For this review, use the dimensioned drawing (mm, ordinates from the lowest corner) and the shaded views. A direction names the side the tool comes from. Coordinates: 2 decimals unless noted, no trailing zeros. Loops run counter-clockwise (first coordinate to the right, second up) from the corner with the lowest first, then second, coordinate; pieces in that order, holes last. Notation, with made-up numbers: M -34,-17.5 L 13,-17.5 A24 ccw 13,16.5 Z; hole C -3,11.25 d8. An arc over 180 degrees is marked long. One line per item, written item: value.
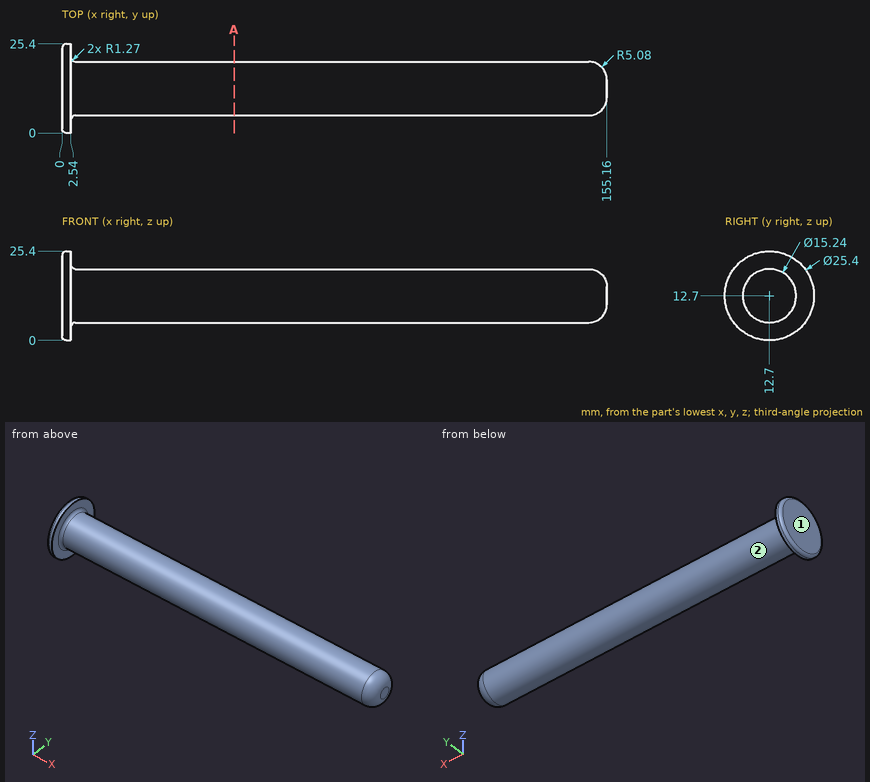
(1) We need section A-A on x = 49. State the section outline as (y, z) points.
Reply:
outline: C 12.7,12.7 d15.24
(2) Tool access review of the marked faces 1 and 2: name each direction out of +Z, -Z, +X, -X, +Y, -Y from which nothing blocks a thin tool from reaching the whole face with its end or side.
Reply:
face 1: +Z, -Z, -X, +Y, -Y
face 2: +X
(3) Insertion check: pin 1 (8 mm diameter, centred on x = 57, z = 20, fed in from +Y); pin 2 (1 mm diameter, centred on x = 26.5, z = 14, fed in from -Y); pin 3 (1.5 mm diameter, centred on x = 114.5, z = 10, fed in from -Y). Each pin has a flat end and moves straight along its axis. Give the tip position at first contact, or say it passes through.
Reply:
pin 1: stops at y = 19.57
pin 2: stops at y = 5.12
pin 3: stops at y = 5.33
(4) To check wall thickness, follow line 1 along X through (y, z) = (15, 23.5); line 2 along Z through (x, y) = (94, 13); line 3 along Y through (x, z) = (38.5, 13.5). State the ranges of each line that lie inside material, in increasing order. Write a range as [from, to].
Reply:
line 1: x = [0, 2.54]
line 2: z = [5.09, 20.31]
line 3: y = [5.12, 20.28]
